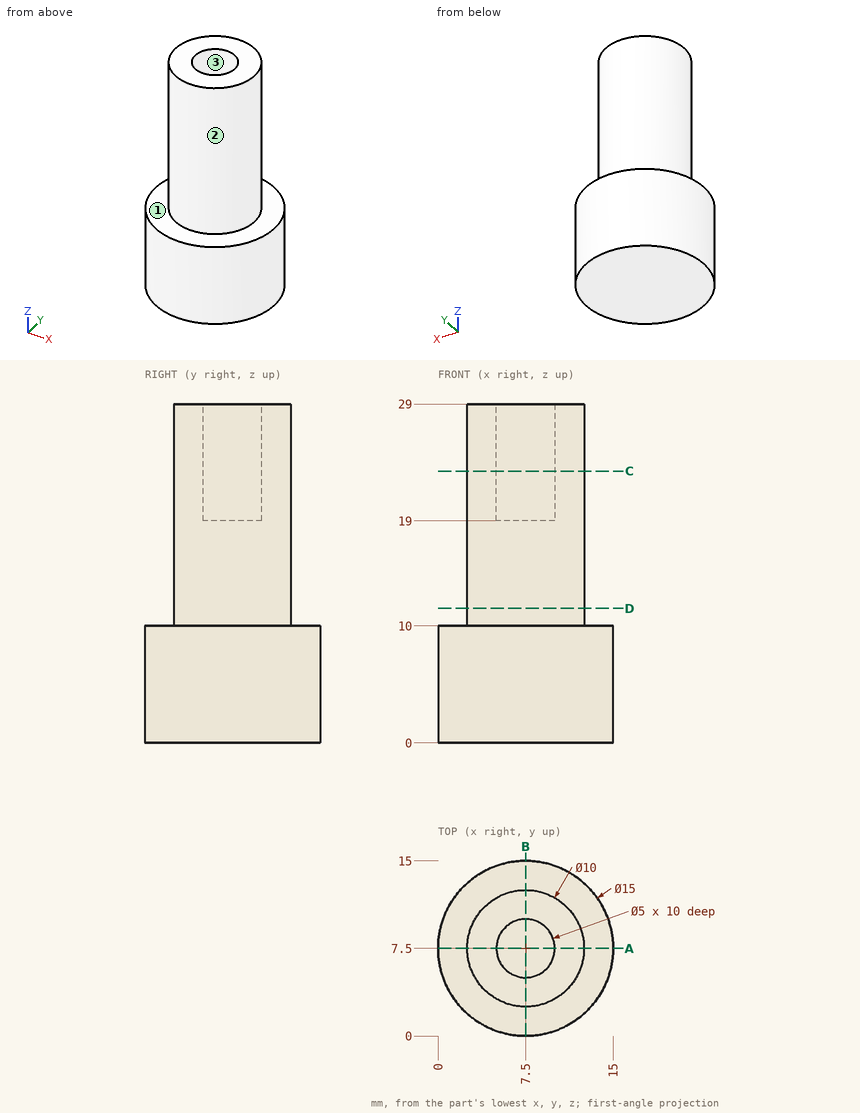
Input: dimensioned drawing with shaded views. Units: mm. Origin: part minimum x, y, z. Round coordinates to 2 decimals unless told otherwise and drop trailing zeros. Order: outer loops, then holes, each group sorted by start corner. A loop starts at its lowest first (then second) coordinate and runs counter-clockwise, first axis right, second up. Notation, with made-up numbers: (53.25, 37.25) -> (101.25, 37.25) arc R27 ccw to (101.25, 58.25) -> close; hole circle Ø3 at (46, -39.5). An arc over 180 degrees is marked (long way). One line per item, written item: value. Start each with the question number.
Q1. Section query D-D (z = 11.5). Return the cut outline in (x, y).
Q2. Material intervals for probe 1 along Y at (x, z) = (7.5, 23.25); probe 2 along Z at (x, y) = (6.5, 13.75); probe 3 along Z at (x, y) = (8, 6), sorted ascending.
Q3. Pin query (flat end, axial travel): pin 1 (3 mm diameter, centred on y = 3.5, z = 9, fed in from +X); pin 2 (5 mm diameter, centred on y = 8.5, z = 17, fed in from +X); pin 3 (1 mm diameter, centred on y = 9.5, z = 13, fed in from -X). Return the tip coordinate at first contact, or that it passes through.
Q4. Section query C-C (z = 23.25). Return the cut outline in (x, y), plus the area to 3 significant figures.
Q5. Draft query along Y for the marked faces 1, 2 and 3. Return one class per face: pulls with the +Y half, pulls with the -Y half, needs draft (parallel to the pull), parting line crosses it, or undercut.
Q6. Section query A-A (y = 7.5). Return the cut outline in (x, z), plus the area to 3 significant figures.
Findings below:
1. outline: circle Ø10 at (7.5, 7.5)
2. probe 1: 2.5 to 5, 10 to 12.5
2. probe 2: 0 to 10
2. probe 3: 0 to 19
3. pin 1: x = 14.57
3. pin 2: x = 12.5
3. pin 3: x = 2.73
4. outline: circle Ø10 at (7.5, 7.5); hole circle Ø5 at (7.5, 7.5)
4. area: 58.9 mm²
5. face 1: needs draft
5. face 2: parting line crosses it
5. face 3: undercut
6. outline: (0, 0) -> (15, 0) -> (15, 10) -> (12.5, 10) -> (12.5, 29) -> (10, 29) -> (10, 19) -> (5, 19) -> (5, 29) -> (2.5, 29) -> (2.5, 10) -> (0, 10) -> close
6. area: 290 mm²
